Geometry check sheet. Reference: drawing and pictorial views, mm from the part's lowest x, y, z. A direction names the side the tool comes from. Coordinates: 2 decimals unless noted, no trailing zeros. Order: outer loops, then holes, each group sorted by start corner. A loop starts at its lowest first (then second) coordinate and runs counter-clockwise, first axis right, second up. Notation, with made-up numbers: M 79,65 L 109,65 A18 cw 109,76 Z; hole C 34,56 d10. An arc over 180 degrees is marked long. Return JSON: item names as keys, results as strings.
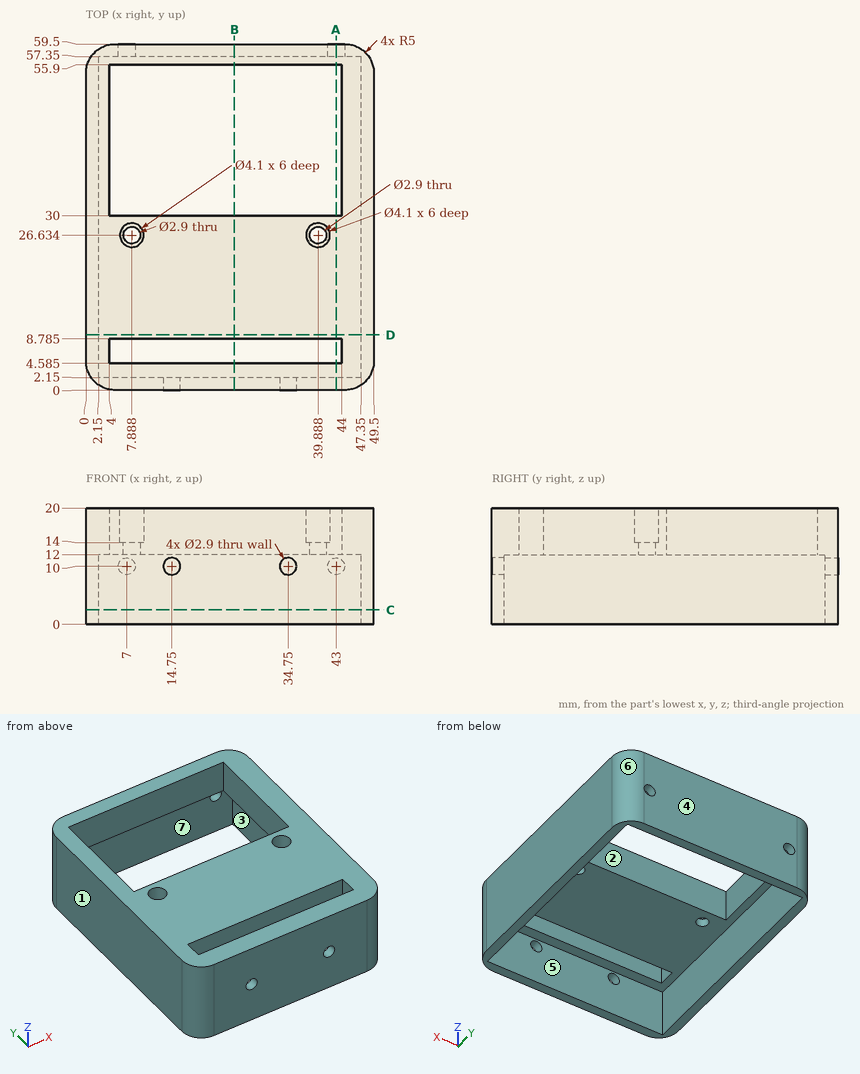
Q1. Cross-section at C-C, the plane z = 2.5. Record the boundary of the cut face in (x, y).
Values:
{"outline": "M 0,5 A5 ccw 5,0 L 44.5,0 A5 ccw 49.5,5 L 49.5,54.5 A5 ccw 44.5,59.5 L 5,59.5 A5 ccw 0,54.5 Z; hole M 2.15,2.15 L 47.35,2.15 L 47.35,57.35 L 2.15,57.35 Z"}
Q2. Go/stop test with flat-tipped pins: pin 1 (2 mm diameter, centred on x = 40, y = 27.5, fed in from +Z); pin 2 (2.5 mm diameter, centred on x = 34.75, z = 10, fed in from -Y); pin 3 (3.5 mm diameter, centred on x = 7.888, y = 26.634, fed in from -Z); pin 4 (4 mm diameter, centred on x = 15.5, y = 53, fed in from -Z). Record where each tip stops, or that it passes through.
Values:
{"pin 1": "z = 14", "pin 2": "y = 57.35", "pin 3": "z = 12", "pin 4": "through"}
Q3. Draft check along X on the marked faces 4, 5, 6 and 7. Enter one of: pulls with the +X half, pulls with the -X half, needs draft (parallel to the pull), parting line crosses it, or undercut.
Values:
{"face 4": "needs draft", "face 5": "undercut", "face 6": "pulls with the +X half", "face 7": "undercut"}
Q4. Cross-section at B-B, the plane x = 25.5. Record the boundary of the cut face in (y, z) (3 decimals).
Values:
{"outline": "M 0,0 L 2.15,0 L 2.15,12 L 4.585,12 L 4.585,20 L 0,20 Z; M 8.785,12 L 30,12 L 30,20 L 8.785,20 Z; M 55.9,12 L 57.35,12 L 57.35,0 L 59.5,0 L 59.5,20 L 55.9,20 Z"}
Q5. Material ranges on line 1 along Y through (x, z) = (37.5, 12.5) (3 decimals); line 2 along Z through (x, y) = (7, 57.8); line 3 along Y through (x, z) = (32, 11), recorded low to high.
Values:
{"line 1": "0 to 4.585, 8.785 to 30, 55.9 to 59.5", "line 2": "0 to 8.55, 11.45 to 20", "line 3": "0 to 2.15, 57.35 to 59.5"}
Q6. Tool access check on the marked faces 1, 2 and 3. Record the directions out of +Z, -Z, +X, -X, +Y, -Y that give a thin tool (end or side, any length) a straight path to the whole face; none if there is none.
Values:
{"face 1": "+Z, -Z, -X, +Y, -Y", "face 2": "+Z, -Z", "face 3": "-Z"}
Q7. Cross-section at A-A, the plane x = 43. Record the boundary of the cut face in (y, z) (3 decimals).
Values:
{"outline": "M 0,0 L 2.15,0 L 2.15,12 L 4.585,12 L 4.585,20 L 0,20 Z; M 8.785,12 L 30,12 L 30,20 L 8.785,20 Z; M 55.9,12 L 57.35,12 L 57.35,11.45 L 59.5,11.45 L 59.5,20 L 55.9,20 Z; M 57.35,0 L 59.5,0 L 59.5,8.55 L 57.35,8.55 Z"}
Q8. Cross-section at D-D, the plane y = 9.5. Record the boundary of the cut face in (x, z).
Values:
{"outline": "M 0,0 L 2.15,0 L 2.15,12 L 47.35,12 L 47.35,0 L 49.5,0 L 49.5,20 L 0,20 Z"}
